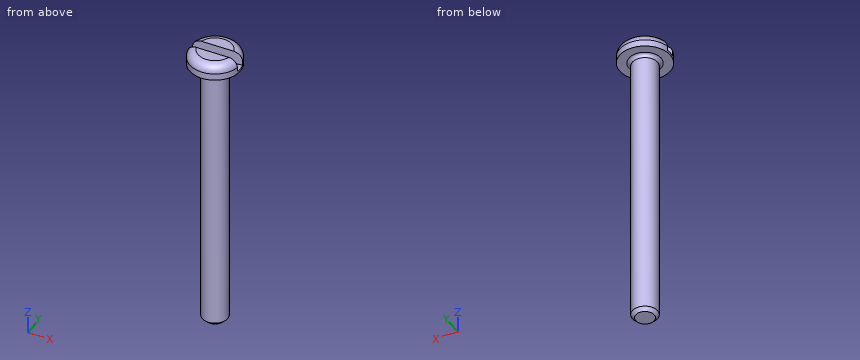
from build123d import *

# Parameters (mm, degrees)
SKETCH_2_W               = 1.5
SKETCH_2_H               = 1.2
CUT_EXTRUDE_1_DEPTH      = 4
CUT_EXTRUDE_1_DEPTH_BACK = 4
CHAMFER_1_SIZE           = 0.4
FILLET_1_R               = 1
FILLET_2_R               = 0.4


with BuildPart() as part:
    # Эскиз1 → Повернуть1 (revolve)
    with BuildSketch(Plane(origin=(0, 0, 0), x_dir=(1, 0, 0), z_dir=(0, 1, 0))):
        Polygon((0, 0), (-3, 0), (-3, 1.8), (-1.5, 1.8), (-1.5, 35), (0, 35), align=None)
    revolve(axis=Axis((0, 0, -35), (0, 0, 1)))

    # Эскиз2 → Вырез-Вытянуть1 (cut, two sides)
    with BuildSketch(Plane(origin=(0, 0, 0), x_dir=(0, 0, -1), z_dir=(1, 0, 0))) as cut_extrude_1_sk:
        with Locations((0.75, 0)):
            Rectangle(SKETCH_2_W, SKETCH_2_H)
    extrude(amount=CUT_EXTRUDE_1_DEPTH, mode=Mode.SUBTRACT)
    extrude(cut_extrude_1_sk.sketch, amount=-CUT_EXTRUDE_1_DEPTH_BACK, mode=Mode.SUBTRACT)

    # Фаска1
    chamfer_1_edges = [part.edges().sort_by_distance(p)[0] for p in [
        (1.5, 0, -35),
    ]]
    chamfer(chamfer_1_edges, length=CHAMFER_1_SIZE)

    # Скругление1
    fillet_1_edges = [part.edges().sort_by_distance(p)[0] for p in [
        (0, 3, 0),
        (0, -3, 0),
    ]]
    fillet(fillet_1_edges, radius=FILLET_1_R)

    # Скругление2
    fillet_2_edges = [part.edges().sort_by_distance(p)[0] for p in [
        (1.5, 0, -1.8),
    ]]
    fillet(fillet_2_edges, radius=FILLET_2_R)


solid = part.part
Check sheet for the modelled part. Datum: model origin and axes. Units: mm. Round coordinates to 2 decimals unless told otherwise and drop trailing zeros. Order: outer loops, then holes, each group sorted by start corner. A loop starts at its lowest first (then second) coordinate and runs counter-clockwise, first axis right, second up.
(1) Scan lines: probe 1 along Y at (x, z) = (0.95, -21); probe 2 along X at (y, z) = (0, -16.5); probe 3 along Y at (x, z) = (1.3, -20). Record each from-to range of solid material in increasing order.
(2) Cross-section at B-B, the plane y = 0. Enter the section's corners in (x, z), and give its area (3 significant figures).
(3) Cross-section at C-C, the plane z = -21. Enter the section's corners in (x, y).
(4) Cross-section at A-A, the plane x = 0. Enter the section's corners in (y, z).
(5) Go/stop test with flat-tipped pins: P1, Ø0.8, axis at x = 1, z = -1, coming from the +Y side; P2, Ø2, axis at x = 2.5, y = -2, coming from the +Z side. Record where each tip stops, or that it passes through.
Check sheet entries:
1. probe 1: y = -1.16 to 1.16
1. probe 2: x = -1.5 to 1.5
1. probe 3: y = -0.75 to 0.75
2. outline: (-3, -1.8) - (-1.9, -1.8) arc R0.4 cw to (-1.5, -2.2) - (-1.5, -34.6) - (-1.1, -35) - (1.1, -35) - (1.5, -34.6) - (1.5, -2.2) arc R0.4 cw to (1.9, -1.8) - (3, -1.8) - (3, -1.5) - (-3, -1.5) - close
2. area: 101 mm2
3. outline: circle Ø3 at (0, 0)
4. outline: (-3, -1.8) - (-1.9, -1.8) arc R0.4 cw to (-1.5, -2.2) - (-1.5, -34.6) - (-1.1, -35) - (1.1, -35) - (1.5, -34.6) - (1.5, -2.2) arc R0.4 cw to (1.9, -1.8) - (3, -1.8) - (3, -1) arc R1 ccw to (2, 0) - (0.6, 0) - (0.6, -1.5) - (-0.6, -1.5) - (-0.6, 0) - (-2, 0) arc R1 ccw to (-3, -1) - close
5. P1: stops at y = 2.94
5. P2: stops at z = -0.02
